Part print with two shaded views. Sizes in mm from the minimum x, y, z corner. Round coordinates to 2 decimals unless told otherwise and drop trailing zeros. Loops run counter-clockwise (first coordinate to the right, second up) from the corner with the lowest first, then second, coordinate; pieces in that order, holes last. Notation, with made-up numbers: (5.5, 67) - (21.5, 67) arc R14 ccw to (21.5, 87) - close; hole circle Ø8 at (28, 14.25). An arc over 180 degrees is marked (long way). Use a Markdown table: item, result.
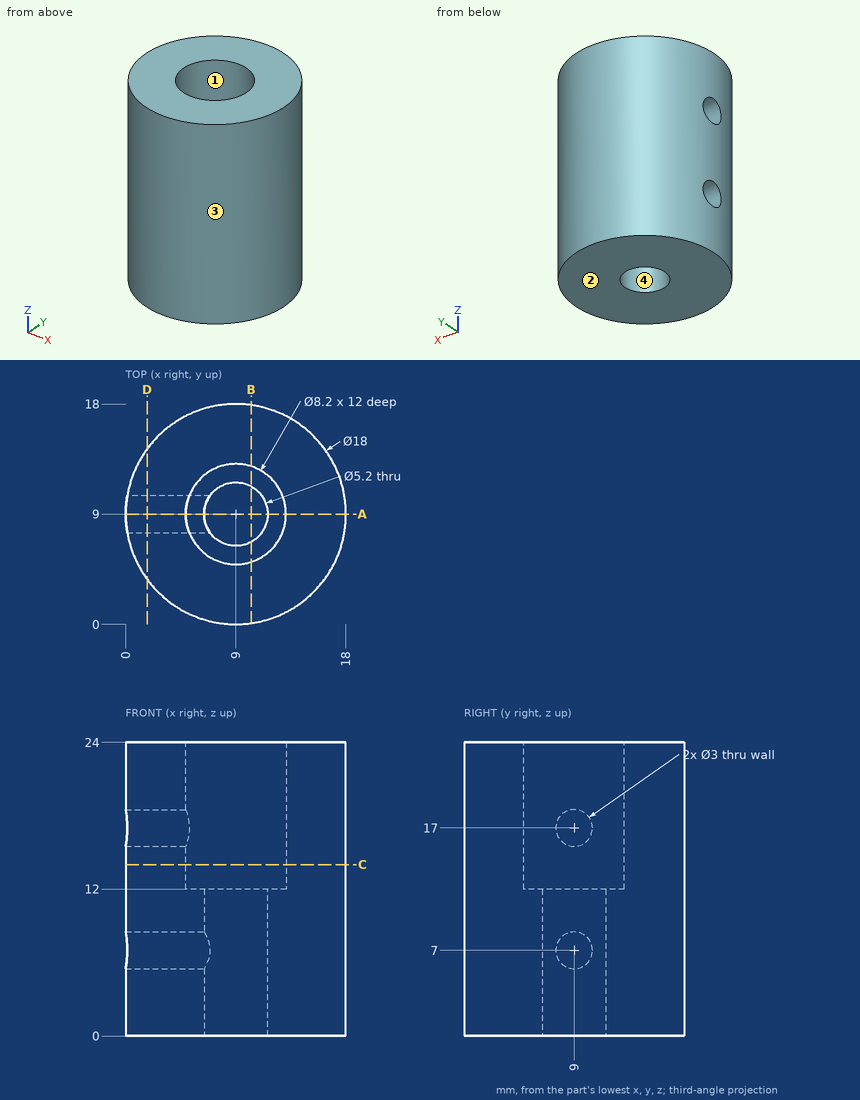
Q1. Cut at D-D, the plane x = 1.75. List the corners of the cut face in (y, z), plus the area to 3 significant figures.
Results found:
| item | result |
|---|---|
| outline | (3.67, 0) - (14.33, 0) - (14.33, 24) - (3.67, 24) - close; hole circle Ø3 at (9, 7); hole circle Ø3 at (9, 17) |
| area | 242 mm2 |
Q2. Cut at A-A, the plane y = 9. List the corners of the cut face in (x, z).
Results found:
| item | result |
|---|---|
| outline | (0, 0) - (6.4, 0) - (6.4, 5.5) - (0, 5.5) - close; (0, 8.5) - (6.4, 8.5) - (6.4, 12) - (4.9, 12) - (4.9, 15.5) - (0, 15.5) - close; (0, 18.5) - (4.9, 18.5) - (4.9, 24) - (0, 24) - close; (11.6, 0) - (18, 0) - (18, 24) - (13.1, 24) - (13.1, 12) - (11.6, 12) - close |
Q3. Cut at C-C, the plane z = 14. List the corners of the cut face in (x, y), plus the area to 3 significant figures.
Results found:
| item | result |
|---|---|
| outline | circle Ø18 at (9, 9); hole circle Ø8.2 at (9, 9) |
| area | 202 mm2 |
Q4. Cut at B-B, the plane x = 10.25. List the corners of the cut face in (y, z), plus the area to 3 significant figures.
Results found:
| item | result |
|---|---|
| outline | (0.09, 0) - (6.72, 0) - (6.72, 12) - (5.1, 12) - (5.1, 24) - (0.09, 24) - close; (11.28, 0) - (17.91, 0) - (17.91, 24) - (12.9, 24) - (12.9, 12) - (11.28, 12) - close |
| area | 279 mm2 |
Q5. Probe line 1 (Z direction, x = 1.25, y = 8); line 2 (Y direction, x = 6.5, z = 19.25); line 3 (Y direction, x = 9.5, z = 2.5). List the from-to ranges inside material, lowest first.
Results found:
| item | result |
|---|---|
| line 1 | z = 0 to 5.88, 8.12 to 15.88, 18.12 to 24 |
| line 2 | y = 0.35 to 5.75, 12.25 to 17.65 |
| line 3 | y = 0.01 to 6.45, 11.55 to 17.99 |
Q6. Pull direction Y, two halves, no side cores. Call the marked faces 1, 2, 3 and 4: pulls with the +Y half, pulls with the -Y half, needs draft (parallel to the pull), parting line crosses it, or undercut.
Results found:
| item | result |
|---|---|
| face 1 | undercut |
| face 2 | needs draft |
| face 3 | parting line crosses it |
| face 4 | undercut |
Q7. Drop flat-ended pins along their axis: pin 1 (3 mm diameter, centred on x = 11.5, z = 14.5, fed in from -Y); pin 2 (4 mm diameter, centred on x = 8.5, y = 7.5, fed in from +Z); pin 3 (1 mm diameter, centred on y = 5.5, z = 21, fed in from -X). Give the stop position or say it passes through.
Results found:
| item | result |
|---|---|
| pin 1 | stops at y = 0.06 |
| pin 2 | stops at z = 12 |
| pin 3 | stops at x = 0.51 |
